Input: part model. Units: mm. Frame: model coordinates. Give positions to 0.01 mm unless a question says otherwise; leave off trailing zeros. Loops run counter-clockwise (first coordinate to the right, second up) from the corner with the lowest first, then second, coordinate; pieces in that order, holes last.
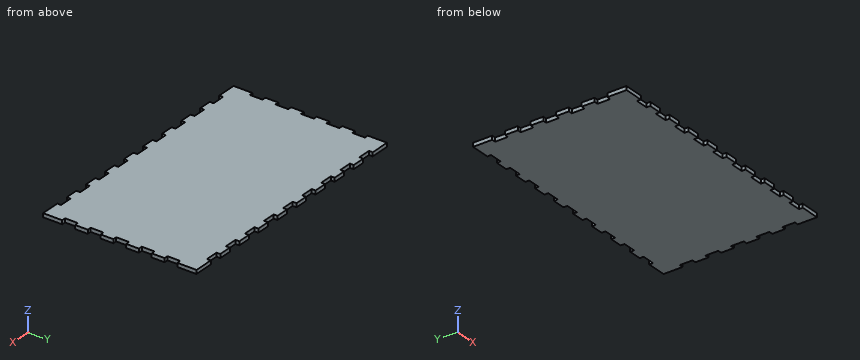
from build123d import *

# Parameters (mm, degrees)
F0_W     = 400
F0_H     = 240
F1_DEPTH = 6
F2_W     = 6
F2_H     = 20
F2_W_2   = 20
F2_H_2   = 6
F3_DEPTH = 25


with BuildPart() as f1:
    # F0 (on Top) → F1 (new body)
    with BuildSketch(Plane.XY):
        Rectangle(F0_W, F0_H)
    extrude(amount=F1_DEPTH)

    # F2 (on face) → F3 (cut)
    with BuildSketch(Plane.XY.offset(6)):
        with Locations((-197, 80)):
            Rectangle(F2_W, F2_H)
        with Locations((-197, 40)):
            Rectangle(F2_W, F2_H)
        with Locations((-197, -40)):
            Rectangle(F2_W, F2_H)
        with Locations((-197, 0)):
            Rectangle(F2_W, F2_H)
        with Locations((-197, -80)):
            Rectangle(F2_W, F2_H)
        with Locations((-160, 117)):
            Rectangle(F2_W_2, F2_H_2)
        with Locations((-120, 117)):
            Rectangle(F2_W_2, F2_H_2)
        with Locations((-80, 117)):
            Rectangle(F2_W_2, F2_H_2)
        with Locations((-40, 117)):
            Rectangle(F2_W_2, F2_H_2)
        with Locations((0, 117)):
            Rectangle(F2_W_2, F2_H_2)
        with Locations((40, 117)):
            Rectangle(F2_W_2, F2_H_2)
        with Locations((80, 117)):
            Rectangle(F2_W_2, F2_H_2)
        with Locations((120, 117)):
            Rectangle(F2_W_2, F2_H_2)
        with Locations((160, 117)):
            Rectangle(F2_W_2, F2_H_2)
        with Locations((197, 80)):
            Rectangle(F2_W, F2_H)
        with Locations((197, 40)):
            Rectangle(F2_W, F2_H)
        with Locations((197, 0)):
            Rectangle(F2_W, F2_H)
        with Locations((197, -40)):
            Rectangle(F2_W, F2_H)
        with Locations((197, -80)):
            Rectangle(F2_W, F2_H)
        with Locations((-160, -117)):
            Rectangle(F2_W_2, F2_H_2)
        with Locations((-120, -117)):
            Rectangle(F2_W_2, F2_H_2)
        with Locations((-80, -117)):
            Rectangle(F2_W_2, F2_H_2)
        with Locations((-40, -117)):
            Rectangle(F2_W_2, F2_H_2)
        with Locations((0, -117)):
            Rectangle(F2_W_2, F2_H_2)
        with Locations((40, -117)):
            Rectangle(F2_W_2, F2_H_2)
        with Locations((80, -117)):
            Rectangle(F2_W_2, F2_H_2)
        with Locations((120, -117)):
            Rectangle(F2_W_2, F2_H_2)
        with Locations((160, -117)):
            Rectangle(F2_W_2, F2_H_2)
    extrude(amount=-F3_DEPTH, mode=Mode.SUBTRACT)


solid = f1.part
(1) Cut plane B-B (y = 1). Return the cut outline in (x, z).
Values follow:
outline: (-194, 0) - (194, 0) - (194, 6) - (-194, 6) - close
(2) Cut plane A-A (x = 76). Return the cut outline in (y, z), and give its area (3 significant figures).
Values follow:
outline: (-114, 0) - (114, 0) - (114, 6) - (-114, 6) - close
area: 1,370 mm2
(3) Ray query, probe 1 along X at (y, z) = (-34.5, 2); probe 2 along Y at (x, z) = (-83.5, 0.4). Return the intervals inside material, ascending.
Values follow:
probe 1: x = -194 to 194
probe 2: y = -114 to 114
(4) Pin query (flat end, axial travel): pin 1 Ø12 at (x, y) = (127.5, -40) entering from -Z; pin 2 Ø1.8 at (y, z) = (41.5, 3) entering from -X; pin 3 Ø3 at (y, z) = (38, 3) entering from +X. Return the tip coordinate at first contact, or that it passes through.
Values follow:
pin 1: stops at z = 0
pin 2: stops at x = -194
pin 3: stops at x = 194
